```python
from build123d import *

# Parameters (mm, degrees)
SKETCH_R     = 4.5
SKETCH_R_2   = 3.5
PAD_DEPTH    = 10
SKETCH001_R  = 7.5
PAD001_DEPTH = 3
CHAMFER_SIZE = 2.99
SKETCH003_W  = 2
SKETCH003_H  = 10
POCKET_DEPTH = 6
FILLET_R     = 0.5
FILLET001_R  = 0.3


with BuildPart() as part:
    # Sketch (on XY_Plane of Origin) → Pad (new body)
    with BuildSketch(Plane.XY):
        Circle(SKETCH_R)
        Circle(SKETCH_R_2, mode=Mode.SUBTRACT)
    extrude(amount=PAD_DEPTH)

    # Sketch001 (on XY_Plane of Origin) → Pad001 (join)
    with BuildSketch(Plane.XY):
        Circle(SKETCH001_R)
    extrude(amount=PAD001_DEPTH)

    # Chamfer
    chamfer_edges = [part.edges().sort_by_distance(p)[0] for p in [
        (-7.5, 0, 3),
    ]]
    chamfer(chamfer_edges, length=CHAMFER_SIZE)

    # Sketch002 (on YZ_Plane of Origin) → Revolution (revolve)
    with BuildSketch(Plane.YZ):
        Polygon((4.1, 8.7), (4.706218, 8.35), (4.1, 8), align=None)
    revolve(axis=Axis((0, 0, 0), (0, 0, 1)))

    # Sketch003 (on YZ_Plane of Origin) → Pocket (cut, symmetric)
    with BuildSketch(Plane.YZ):
        with Locations((0, 8)):
            Rectangle(SKETCH003_W, SKETCH003_H)
    extrude(amount=POCKET_DEPTH, both=True, mode=Mode.SUBTRACT)

    # Fillet
    fillet_edges = [part.edges().sort_by_distance(p)[0] for p in [
        (0, -3.5, 3),
        (0, 3.5, 3),
        (3.870792, 1, 3),
        (-3.870792, 1, 3),
        (3.870792, -1, 3),
        (-3.870792, -1, 3),
    ]]
    fillet(fillet_edges, radius=FILLET_R)

    # Fillet001
    fillet001_edges = [part.edges().sort_by_distance(p)[0] for p in [
        (0, 4.5, 10),
        (0, -4.5, 10),
    ]]
    fillet(fillet001_edges, radius=FILLET001_R)


solid = part.part
```
Could you check a few things on this model? Use its own coordinates, in mm. A direction names the side the tool comes from. Round coordinates to 2 decimals unless told otherwise and drop trailing zeros. Order: outer loops, then holes, each group sorted by start corner. A loop starts at its lowest first (then second) coordinate and runs counter-clockwise, first axis right, second up. Notation, with made-up numbers: M -17.5,56 L -4.5,56 A16 cw -4.5,67 Z; hole C -6,-13.75 d4. An arc over 180 degrees is marked long. One line per question, with ' | ' between items. Start each with the question number.
(1) Suppose I cut it at A-A on z = 4. List the corners of the cut face in (x, y) for me, then the cut area to 3 significant figures.
(2) For faces 1 (the face through (0.1, 4.5, 5.6)), 2 (the face through (0.1, 3.5, 6.7)), 3 (the face through (-0.1, -4.5, 9.1)), 4 (the face through (4, -1, 7)), which set-ups out of +Z, -Z, +X, -X, +Y, -Y let a thin tool reach every point of the face, with its end or its side?
(3) Please list where these lines run through material, in increasing order: line 1 along Y through (x, z) = (-4.5, 1); line 2 along Y through (x, z) = (-1.75, 4.75); line 3 along X through (y, z) = (-2.5, 9).
(4) For P1, Ø1.4, axis at x = -4, z = 5, coming from the -Y side; P2, Ø1.5, axis at x = -0.5, y = 5.5, coming from the +Z side; P3, Ø1.5, axis at x = -0.5, z = 4.5, coming from the +Y side, each with a flat end and sliding along its axis, tell me the tip position at first contact or that it passes through.
(5) Suppose I cut it at D-D on z = 1.75. List the corners of the cut face in (x, y) for me, then the cut area to 3 significant figures.
(6) Thinking about a two-plate mould opening in Z: for faces 5 (the face through (-0.1, -4.5, 5.6)), 6 (the face through (-4, 1, 7)), 7 (the face through (0, 0, 0)), which applies, +Z half, -Z half, draft (parallel to the pull), parting line (faces both ways), or undercut?
Geometry results:
1) outline: M -4.39,-1 A4.5 ccw 4.39,-1 L 3.35,-1 A3.5 cw -3.35,-1 Z; M -4.39,1 L -3.35,1 A3.5 cw 3.35,1 L 4.39,1 A4.5 ccw Z | area: 21.1 mm²
2) face 1: +Y | face 2: +Z | face 3: +Z, -Y | face 4: +Z, +X, -X
3) line 1: -4.7 to 4.7 | line 2: -4.15 to -3.03, 3.03 to 4.15 | line 3: -3.74 to -2.45, 2.45 to 3.74
4) P1: y = -3.06 | P2: z = 2.74 | P3: y = 4.5
5) outline: C 0,0 d11.52 | area: 104 mm²
6) face 5: undercut | face 6: draft | face 7: -Z half
